Here's how the part is built. I have some questions about the finished solid (model axes, mm). A direction names the side the tool comes from. Coordinates: 2 decimals unless noted, no trailing zeros. Write each loop counter-clockwise with the first axis right and the second up, starting at its lowest first coordinate (ties: lowest second). Pieces come first, ordered by that corner, then holes.
(1) For pin 1 Ø1 at (x, y) = (-52.5, -42.5) entering from -Z; pin 2 Ø8 at (x, y) = (100.5, 7) entering from +Z; pin 3 Ø3 at (y, z) = (-29, -48.5) entering from +X, each with a flat end and sliding along its axis, tell me the tip position at first contact or that it passes through.
(2) Imagine slicing it at C-C, the plane x = 50. List the corners of the cut face in (y, z) for me, plus the area to 3 significant figures.
(3) Thinking about a two-plate mould opening in X: for faces 1 (the flat face through (135.128, 1, 1)), 2 (the flat face through (64.77, -27, 1)), 3 (the cylindrical face through (55.76, -13.49, -60.75)), 4 (the flat face through (-135.128, -1, 1)), which applies, released by +X, released by -X, zero draft, split by the parting line, or undercut?
(4) Please list where these lines run through material, in increasing order: probe 1 along X at (y, z) = (30, 10); probe 2 along X at (y, z) = (57, 17.5); probe 3 along X at (y, z) = (29.5, 38).
(5) Which directions (+Z, -Z, +X, -X, +Y, -Y) give clear straight access to the entire face, cutting with the end or side of a thin tool? Please do faces 5 (the cylindrical face through (-133.25, -38.9, -29.83)), 6 (the cylindrical face through (-56, -13.49, -60.75)), 7 (the cylindrical face through (133.2, -38.9, -29.83)), 8 (the flat face through (-64.77, 27, 1)).
(6) Imagine slicing it at D-D, the plane z = -29. State how many separate pieces and enclosed holes the cut face has, plus the area to 3 significant figures.
```python
from build123d import *


with BuildPart() as part:
    # Sketch1 → Revolve1 (revolve)
    with BuildSketch(Plane.XY):
        Polygon((-135.128, 49.022), (-135.128, 0), (0, 0), (0, 25.4), (-46.99, 25.4), (-46.99, 62.23), (-64.77, 62.23), (-64.77, 25.4), (-128.778, 25.4), (-128.778, 46.482), (-131.318, 49.022), align=None)
        Polygon((0, 25.4), (0, 0), (135.128, 0), (135.128, 49.022), (131.318, 49.022), (128.778, 46.482), (128.778, 25.4), (64.77, 25.4), (64.77, 62.23), (46.99, 62.23), (46.99, 25.4), align=None)
    revolve(axis=Axis((-135.128, 0, 0), (1, 0, 0)))


solid = part.part
```
Recorded:
1. pin 1: stops at z = -45.92
1. pin 2: stops at z = 25.22
1. pin 3: stops at x = 64.77
2. outline: circle Ø124.46 at (0, 0)
2. area: 12,200 mm2
3. face 1: released by +X
3. face 2: undercut
3. face 3: zero draft
3. face 4: released by -X
4. probe 1: x = -135.13 to -128.78, -64.77 to -46.99, 46.99 to 64.77, 128.78 to 135.13
4. probe 2: x = -64.77 to -46.99, 46.99 to 64.77
4. probe 3: x = -135.13 to -130.4, -64.77 to -46.99, 46.99 to 64.77, 130.4 to 135.13
5. face 5: -X
5. face 6: +X, -X
5. face 7: +X
5. face 8: none
6. separate pieces: 4
6. enclosed holes: 0
6. area: 4,900 mm2
